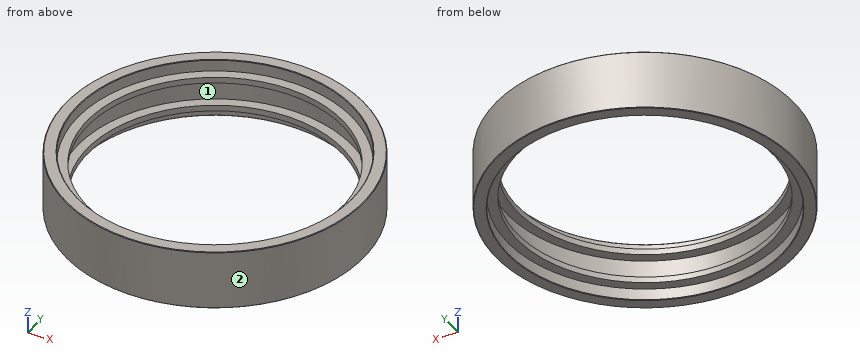
```python
from build123d import *

# Parameters (mm, degrees)
SMUSSO1_SIZE = 0.05


with BuildPart() as part:
    # Schizzo2 → Rivoluzione1 (revolve)
    with BuildSketch(Plane(origin=(0, 0, 0), x_dir=(0, 0, -1), z_dir=(1, 0, 0))):
        Polygon((0.563380282, 12.5), (5.563380282, 12.5), (5.563380282, 11.5), (4.563380282, 11.5), (4.563380282, 10.7), (4.063380282, 10.7), (4.063380282, 11.5), (2.063380282, 11.5), (2.063380282, 10.7), (1.563380282, 10.7), (1.563380282, 11.5), (0.563380282, 11.5), align=None)
    revolve(axis=Axis((0, 0, 0), (0, 0, 1)))

    # Smusso1
    smusso1_edges = [part.edges().sort_by_distance(p)[0] for p in [
        (0, -11.5, -5.563380282),
        (0, -12.5, -5.563380282),
        (0, -12.5, -0.563380282),
        (0, -11.5, -0.563380282),
    ]]
    chamfer(smusso1_edges, length=SMUSSO1_SIZE)


solid = part.part
```
Can you work these out from the model? Positions are in its coordinate system, mm. Face numbers are marked on the shaded views. Give positions to 0.01 mm unless a question says otherwise; leave off trailing zeros. Loops run counter-clockwise (first coordinate to the right, second up) from the corner with the lowest first, then second, coordinate; pieces in that order, holes last. Notation, with made-up numbers: M 31,25 L 63,25 A31 ccw 63,57 Z; hole C 34,-8.75 d4. An arc over 180 degrees is marked long. Use one line per item in the form item = value. Start each with the question number.
(1) I want a section at C-C, the plane z = -0.9. Write out the boundary of the cut face in (x, y), and give its area (3 significant figures).
(2) Please list where these lines run through material, in increasing order: line 1 (Y direction, x = 0, z = -2.8); line 2 (Y direction, x = 0, z = -1.85).
(3) Thinking about a two-plate mould opening in X: for the marked faces 1 and 2, which applies, released by +X, released by -X, zero draft, split by the parting line, or undercut?
(4) I'm going to push flat-ended pins straight in: P1, Ø5, axis at x = 3.5, y = -5.5, coming from the -Z side; P2, Ø2, axis at x = 3.5, y = -9.5, coming from the +Z side; P3, Ø3, axis at x = -6, z = -5, coming from the +Y side. Where does each tip first touch, or does it pass through?
Worked out:
q1.outline = C 0,0 d25; hole C 0,0 d23
q1.area = 75.4 mm²
q2.line_1 = -12.5 to -11.5, 11.5 to 12.5
q2.line_2 = -12.5 to -10.7, 10.7 to 12.5
q3.face_1 = undercut
q3.face_2 = split by the parting line
q4.P1 = through
q4.P2 = -1.56
q4.P3 = 11.66
